Read the model definition and answer for the solid it produces. Units are mm, in the model's axes. A direction names the side the tool comes from. Give positions to 0.01 mm unless a question says otherwise; leave off trailing zeros. Order: outer loops, then holes, each group sorted by start corner. A loop starts at its lowest first (then second) coordinate and runs counter-clockwise, first axis right, second up. Notation, with made-up numbers: M -27.75,43.5 L -9.75,43.5 A22 ccw -9.75,74.5 Z; hole C 7.5,60.5 d10. An arc over 180 degrees is marked long. One line per item, written item: value.
from build123d import *

# Parameters (mm, degrees)
F1_DEPTH = 2
F2_R     = 5


with BuildPart() as f1:
    # F0 (on Top) → F1 (new body)
    with BuildSketch(Plane.XY):
        with BuildLine():
            Line((-4, 12.71492), (-4, 0))
            Line((-4, 0), (0, 0))
            Line((0, 0), (4, 0))
            Line((4, 0), (4, 12.71492))
            ThreePointArc((4, 12.71492), (2.861128, 30.04824), (5.073318, 47.277495))
            Line((5.073318, 47.277495), (1.460623, 116.211824))
            Line((1.460623, 116.211824), (0, 120.224852))
            Line((0, 120.224852), (-1.460623, 116.211824))
            Line((-1.460623, 116.211824), (-5.073318, 47.277495))
            ThreePointArc((-5.073318, 47.277495), (-2.861128, 30.04824), (-4, 12.71492))
        make_face()
    extrude(amount=F1_DEPTH)

    # F2
    f2_edges = [f1.edges().sort_by_distance(p)[0] for p in [
        (-1.460623, 116.211824, 1),
        (1.460623, 116.211824, 1),
        (5.073318, 47.277495, 1),
        (-5.073318, 47.277495, 1),
        (-4, 12.71492, 1),
        (4, 12.71492, 1),
    ]]
    fillet(f2_edges, radius=F2_R)


solid = f1.part
1) Find section B-B, the plane y = 84. Write down the section's boundary in (x, z), plus the area to 3 significant figures.
Reported:
outline: M -3.15,0 L 3.15,0 L 3.15,2 L -3.15,2 Z
area: 12.6 mm^2
2) Which of the six approach directions +Z, -Z, +X, -X, +Y, -Y give full straight-line access (tool end or side, diameter ignored) to faces 5 (the face through (-3.244, 82.187, 0.986)), 6 (the face through (4, 6, 1))?
Reported:
face 5: +Z, -Z, -X, +Y
face 6: +Z, -Z, +X, -Y
3) Consider probe 1 along X at (y, z) = (90.5, 1.4); probe 2 along X at (y, z) = (68.5, 0.5). Determine where each line is inside the solid, lowest interval first.
Reported:
probe 1: x = -2.81 to 2.81
probe 2: x = -3.96 to 3.96
4) Determine the mould class of faces 1 (the face through (2.85, 29.67, 0.99)), 2 (the face through (0, 0, 1)), 3 (the face through (3.293, 81.242, 0.986)), 4 (the face through (-4, 6, 1)) for opening direction Y: +Y half, -Y half, draft (parallel to the pull), parting line (faces both ways), or undercut.
Reported:
face 1: undercut
face 2: -Y half
face 3: +Y half
face 4: draft
5) Find section A-A, the plane z = 0.85. Write down the section's boundary in (x, y).
Reported:
outline: M -5.04,47.96 A5 ccw -4.93,46.63 A90 cw -3.94,13.1 A5 ccw -4,12.31 L -4,0 L 4,0 L 4,12.31 A5 ccw 3.94,13.1 A90 cw 4.93,46.63 A5 ccw 5.04,47.96 L 1.5,115.47 A5 ccw 1.21,116.91 L 0,120.22 L -1.21,116.91 A5 ccw -1.5,115.47 Z
6) Find section C-C, the plane y = 29. Write down the section's boundary in (x, z).
Reported:
outline: M -2.83,0 L 2.83,0 L 2.83,2 L -2.83,2 Z
